Geometry check sheet. Reference: the model listing, model coordinates, mm. A direction names the side the tool comes from. Coordinates: 2 decimals unless noted, no trailing zeros. Order: outer loops, then holes, each group sorted by start corner. A loop starts at its lowest first (then second) coordinate and runs counter-clockwise, first axis right, second up. Notation, with made-up numbers: (54.5, 2.25) - (67.5, 2.25) arc R30 ccw to (67.5, 27.25) - close; hole circle Ø3 at (80.25, 81.5). An arc over 180 degrees is marked (long way). Put each result on its own line as item: value.
from build123d import *

# Parameters (mm, degrees)
BOSS_EXTRUDE1_DEPTH = 6.35
CUT_EXTRUDE1_DEPTH  = 110.933515147


with BuildPart() as part:
    # Sketch1 → Boss-Extrude1 (new body)
    with BuildSketch(Plane(origin=(0, 0, 0), x_dir=(1, 0, 0), z_dir=(0, 1, 0))):
        with BuildLine():
            Line((0, 6.35), (0, 86.286703653))
            ThreePointArc((0, 86.286703653), (-4.706499064, 92.420332649), (-11.849261314, 89.461703653))
            Line((-11.849261314, 89.461703653), (-58.000738686, 9.525))
            ThreePointArc((-58.000738686, 9.525), (-58.000738686, 3.175), (-52.501477372, 0))
            Line((-52.501477372, 0), (-6.35, 0))
            ThreePointArc((-6.35, 0), (-1.859871939, 1.859871939), (0, 6.35))
        make_face()
    extrude(amount=BOSS_EXTRUDE1_DEPTH)

    # Sketch3 → Cut-Extrude1 (cut, through all)
    with BuildSketch(Plane.XZ):
        with BuildLine():
            Line((-23.869488686, -6.604), (-34.981988686, -6.604))
            Line((-34.981988686, -6.604), (-34.981988686, -3.175))
            ThreePointArc((-34.981988686, -3.175), (-35.911924656, -0.92993597), (-38.156988686, 0))
            Line((-38.156988686, 0), (-20.694488686, 0))
            ThreePointArc((-20.694488686, 0), (-22.939552716, -0.92993597), (-23.869488686, -3.175))
            Line((-23.869488686, -3.175), (-23.869488686, -6.604))
        make_face()
    extrude(amount=-CUT_EXTRUDE1_DEPTH, mode=Mode.SUBTRACT)


solid = part.part
Q1. Access from +Z, -Z, +X, -X, +Y, -Y to the whole of each face (thin tool, end or side, straight path). Record for faces 1 (the cylindrical face through (-35.89, 3.13, -0.95)), 2 (the flat face through (-34.602, 3.131, -50.053)).
Answer block:
face 1: +Z, +Y, -Y
face 2: -Z, -X, +Y, -Y
Q2. Thickness scan on L1, parallel to X at y = 4.5, z = -42; L2, parallel to Z at x = -18.5, y = 3.5; L3, parallel to X at y = 4, z = -86. Record the ranges inside material, lowest first. Write a range as [from, to].
Answer block:
L1: x = [-39.25, 0]
L2: z = [-77.94, 0]
L3: x = [-13.85, 0]
Q3. Section check C-C on x = -22. Record the boundary of the cut face in (y, z), then the cut area to 3 significant figures.
Answer block:
outline: (0, -71.88) - (6.35, -71.88) - (6.35, -0.28) - (0, -0.28) - close
area: 455 mm^2
Q4. Depth check by flat-ended pin: pin 1 Ø3 at (x, y) = (-26, 2.5) entering from -Z; pin 2 Ø2.5 at (y, z) = (4.5, -5.5) entering from -X; pin 3 Ø1 at (y, z) = (4, -4.5) entering from +X. Enter the tip coordinate at first touch or a pass-through.
Answer block:
pin 1: stops at z = -67.55
pin 2: stops at x = -58.85
pin 3: stops at x = -0.15
Q5. Section check B-B on z = -41. Record the boundary of the cut face in (x, y).
Answer block:
outline: (-39.83, 0) - (0, 0) - (0, 6.35) - (-39.83, 6.35) - close
Q6. Section check A-A on y = 2.5. Record the boundary of the cut face in (x, z) (3 decimals), then the cut area to 3 significant figures.
Answer block:
outline: (-58.001, -9.525) - (-11.849, -89.462) arc R6.35 ccw to (0, -86.287) - (0, -6.35) arc R6.35 ccw to (-6.35, 0) - (-20.694, 0) arc R3.175 ccw to (-23.869, -3.175) - (-23.869, -6.604) - (-34.982, -6.604) - (-34.982, -3.175) arc R3.175 ccw to (-38.157, 0) - (-52.501, 0) arc R6.35 ccw to start
area: 3,280 mm^2
